from build123d import *

# Parameters (mm, degrees)
F1_DEPTH = 145.542


with BuildPart() as f1:
    # F0 (on Right) → F1 (new body)
    with BuildSketch(Plane.YZ):
        with BuildLine():
            Line((-8.008403, 37.52215), (-8.008403, 0))
            Line((-8.008403, 0), (-8.008403, -37.52215))
            Line((-8.008403, -37.52215), (-18.168403, -37.52215))
            Line((-18.168403, -37.52215), (-18.168403, -32.69615))
            Line((-18.168403, -32.69615), (-21.978403, -32.69615))
            Line((-21.978403, -32.69615), (-21.978403, -34.98215))
            ThreePointArc((-21.978403, -34.98215), (-20.118531, -39.472278), (-15.628403, -41.33215))
            Line((-15.628403, -41.33215), (-10.548403, -41.33215))
            ThreePointArc((-10.548403, -41.33215), (-6.058275, -39.472278), (-4.198403, -34.98215))
            Line((-4.198403, -34.98215), (-4.198403, 0))
            Line((-4.198403, 0), (-4.198403, 34.98215))
            ThreePointArc((-4.198403, 34.98215), (-6.058275, 39.472278), (-10.548403, 41.33215))
            Line((-10.548403, 41.33215), (-15.628403, 41.33215))
            ThreePointArc((-15.628403, 41.33215), (-20.118531, 39.472278), (-21.978403, 34.98215))
            Line((-21.978403, 34.98215), (-21.978403, 32.69615))
            Line((-21.978403, 32.69615), (-18.168403, 32.69615))
            Line((-18.168403, 32.69615), (-18.168403, 37.52215))
            Line((-18.168403, 37.52215), (-8.008403, 37.52215))
        make_face()
    extrude(amount=F1_DEPTH)


solid = f1.part
The model under review builds one solid part; all positions refer to its coordinate system, in mm. A direction names the side the tool comes from. Coordinates: 2 decimals unless noted, no trailing zeros. Loops run counter-clockwise (first coordinate to the right, second up) from the corner with the lowest first, then second, coordinate; pieces in that order, holes last.
(1) Consider section B-B, the plane x = 82. Give the boundary of the cut face in (y, z), plus the area to 3 significant figures.
Determined:
outline: (-21.98, -34.98) arc R6.35 ccw to (-15.63, -41.33) - (-10.55, -41.33) arc R6.35 ccw to (-4.2, -34.98) - (-4.2, 34.98) arc R6.35 ccw to (-10.55, 41.33) - (-15.63, 41.33) arc R6.35 ccw to (-21.98, 34.98) - (-21.98, 32.7) - (-18.17, 32.7) - (-18.17, 37.52) - (-8.01, 37.52) - (-8.01, -37.52) - (-18.17, -37.52) - (-18.17, -32.7) - (-21.98, -32.7) - close
area: 424 mm2
(2) Draft analysis for pull direction Y (two halves, no side actions). For faces 1 (the flat face through (72, -4.198, 0)), 2 (the cylindrical face through (71.75, -20.17, -39.42)), 3 (the flat face through (72, -13, 37.522)), 4 (the flat face through (72, -20, -32.696)), state which applies: +Y half, -Y half, draft (parallel to the pull), parting line (faces both ways), or undercut.
Determined:
face 1: +Y half
face 2: -Y half
face 3: undercut
face 4: draft
(3) Tool access review of faces 5 (the flat face through (72, -18.168, 35)), 6 (the flat face through (145.542, -7, -3)): name each direction out of +Z, -Z, +X, -X, +Y, -Y from which nothing blocks a thin tool from reaching the whole face with its end or side.
Determined:
face 5: +X, -X
face 6: +Z, -Z, +X, +Y, -Y
(4) Consider section C-C, the plane y = -20. Give the boundary of the cut face in (x, z), plus the area to 3 significant figures.
Determined:
outline: (0, -39.59) - (145.54, -39.59) - (145.54, -32.7) - (0, -32.7) - close; (0, 32.7) - (145.54, 32.7) - (145.54, 39.59) - (0, 39.59) - close
area: 2,010 mm2
(5) Consider section A-A, the plane y = -14. Give the boundary of the cut face in (x, z), plus the area to 3 significant figures.
Determined:
outline: (0, -41.33) - (145.54, -41.33) - (145.54, -37.52) - (0, -37.52) - close; (0, 37.52) - (145.54, 37.52) - (145.54, 41.33) - (0, 41.33) - close
area: 1,110 mm2
(6) Consider section D-D, the plane z = 14.5. Give the boundary of the cut face in (x, y).
Determined:
outline: (0, -8.01) - (145.54, -8.01) - (145.54, -4.2) - (0, -4.2) - close
(7) Wall thickness on L1, parallel to Z at x = 118, y = -11; L2, parallel to Y at x = 14.5, z = -30; L3, parallel to Z at x = 18.5, y = -19.25: over which ranges is each line inside the solid? List them lowest first.
Determined:
L1: z = -41.33 to -37.52, 37.52 to 41.33
L2: y = -8.01 to -4.2
L3: z = -40.2 to -32.7, 32.7 to 40.2
(8) Insertion check: P1, Ø4, axis at x = 95.5, z = -36, coming from the +Y side; P2, Ø3, axis at x = 67, y = -20, coming from the +Z side; P3, Ø1.1, axis at x = 56, y = -20.5, coming from the -Z side; P4, Ø2, axis at x = 89, y = -6, coming from the -Z side. Each pin has a flat end and moves straight along its axis. Give the tip position at first contact, or say it passes through.
Determined:
P1: stops at y = -4.2
P2: stops at z = 40.65
P3: stops at z = -39.63
P4: stops at z = -40.25
